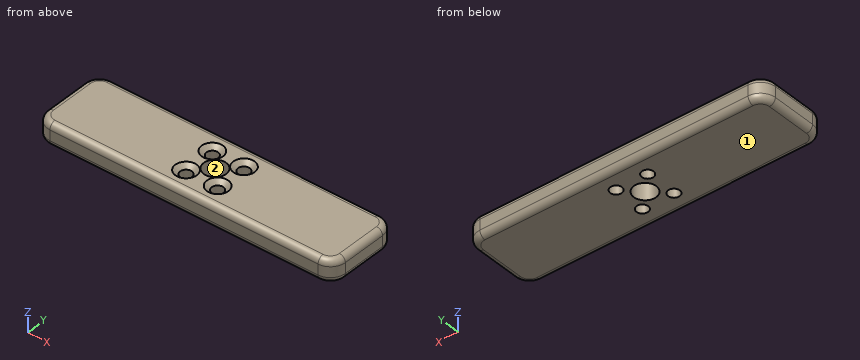
```python
from build123d import *

# Parameters (mm, degrees)
F1_DEPTH        = 9.525
F2_R            = 2.54
F3_R            = 4.7625
F4_DEPTH        = 25.4
F6_D            = 4.9784
F6_CSINK_D      = 9.1186
F6_CSINK_ANGLE  = 100
F6_COPIES_COUNT = 4


# Not quite as in the source:
# - a pattern or mirror of a feature is missing from the dataset's text; its kind, count and spacing are read off the source's solid


with BuildPart() as f1:
    # F0 (on Top) → F1 (new body)
    with BuildSketch(Plane.XY):
        with BuildLine():
            Line((-57.15, -15.875), (57.15, -15.875))
            ThreePointArc((57.15, -15.875), (61.6401280605, -14.0151280605), (63.5, -9.525))
            Line((63.5, -9.525), (63.5, 9.525))
            ThreePointArc((63.5, 9.525), (61.6401280605, 14.0151280605), (57.15, 15.875))
            Line((57.15, 15.875), (-57.15, 15.875))
            ThreePointArc((-57.15, 15.875), (-61.6401280605, 14.0151280605), (-63.5, 9.525))
            Line((-63.5, 9.525), (-63.5, -9.525))
            ThreePointArc((-63.5, -9.525), (-61.6401280605, -14.0151280605), (-57.15, -15.875))
        make_face()
    extrude(amount=F1_DEPTH)

    # F2
    f2_edges = [f1.edges().sort_by_distance(p)[0] for p in [
        (0, -15.875, 9.525),
        (61.640128, -14.015128, 9.525),
        (63.5, 0, 9.525),
        (61.640128, 14.015128, 9.525),
        (0, 15.875, 9.525),
        (-61.640128, 14.015128, 9.525),
        (-63.5, 0, 9.525),
        (-61.640128, -14.015128, 9.525),
        (0, -15.875, 0),
        (61.640128, -14.015128, 0),
        (63.5, 0, 0),
        (61.640128, 14.015128, 0),
        (0, 15.875, 0),
        (-61.640128, 14.015128, 0),
        (-63.5, 0, 0),
        (-61.640128, -14.015128, 0),
    ]]
    fillet(f2_edges, radius=F2_R)

    # F3 (on face) → F4 (cut)
    with BuildSketch(Plane.XY.offset(9.525)):
        Circle(F3_R)
    extrude(amount=-F4_DEPTH, mode=Mode.SUBTRACT)

    # F6 (through all)
    with Locations(Plane.XY.offset(9.525)):
        with Locations((-6.7351920908, 6.7351920908)):
            f6 = CounterSinkHole(F6_D / 2, F6_CSINK_D / 2, counter_sink_angle=F6_CSINK_ANGLE)

    # F6_copies: F6 ×4 about axis
    f6_copies_axis = Axis((0, 0, 0), (0, 0, 1))
    for i in range(1, F6_COPIES_COUNT):
        add(f6.rotate(f6_copies_axis, i * 360 / F6_COPIES_COUNT), mode=Mode.SUBTRACT)


solid = f1.part
```
Could you check a few things on this model? Use its own coordinates, in mm. Face numbers are marked on the shaded views. Coordinates: 2 decimals unless noted, no trailing zeros. Loops run counter-clockwise (first coordinate to the right, second up) from the corner with the lowest first, then second, coordinate; pieces in that order, holes last.
1) Please list where these lines run through material, in increasing order: line 1 along X through (y, z) = (-9, 8); line 2 along X through (y, z) = (9, 2.5); line 3 along Z through (x, y) = (-3, 13.5).
Reported:
line 1: x = -63.29 to -8.28, -5.19 to 5.19, 8.28 to 63.29
line 2: x = -63.5 to -7.77, -5.7 to 5.7, 7.77 to 63.5
line 3: z = 0.01 to 9.52
2) Imagine slicing it at C-C (x = -15). List the corners of the cut face in (y, z) for me (3 decimals).
Reported:
outline: (-15.875, 2.54) arc R2.54 ccw to (-13.335, 0) - (13.335, 0) arc R2.54 ccw to (15.875, 2.54) - (15.875, 6.985) arc R2.54 ccw to (13.335, 9.525) - (-13.335, 9.525) arc R2.54 ccw to (-15.875, 6.985) - close
3) Imagine slicing it at A-A (x = 0). List the corners of the cut face in (y, z) for me (1 decimal), and give its area (3 significant figures).
Reported:
outline: (-15.9, 2.5) arc R2.5 ccw to (-13.3, 0) - (-4.8, 0) - (-4.8, 9.5) - (-13.3, 9.5) arc R2.5 ccw to (-15.9, 7) - close; (4.8, 0) - (13.3, 0) arc R2.5 ccw to (15.9, 2.5) - (15.9, 7) arc R2.5 ccw to (13.3, 9.5) - (4.8, 9.5) - close
area: 206 mm2
4) Imagine slicing it at D-D (z = 5.5). State how many separate pieces and enclosed holes the cut face has, and give its area (3 significant figures).
Reported:
separate pieces: 1
enclosed holes: 5
area: 3,850 mm2
5) Will these pins go through, and if not, where does the flat tip stop? pin 1 Ø5 at (x, z) = (-4, 2) entering from +Y (3 decimals); pin 2 Ø8 at (x, y) = (6.74, 6.74) entering from +Z; pin 3 Ø5.5 at (x, y) = (-6.74, -6.74) entering from +Z.
Reported:
pin 1: stops at y = 15.875
pin 2: stops at z = 9.06
pin 3: stops at z = 8.01
6) Imagine slicing it at B-B (y = 0). List the corners of the cut face in (x, z) for me (1 decimal).
Reported:
outline: (-63.5, 2.5) arc R2.5 ccw to (-61, 0) - (-4.8, 0) - (-4.8, 9.5) - (-61, 9.5) arc R2.5 ccw to (-63.5, 7) - close; (4.8, 0) - (61, 0) arc R2.5 ccw to (63.5, 2.5) - (63.5, 7) arc R2.5 ccw to (61, 9.5) - (4.8, 9.5) - close
7) Thinking about a two-plate mould opening in Y: for the marked faces 1 and 2, which applies, released by +Y, released by -Y, zero draft, split by the parting line, or undercut?
Reported:
face 1: zero draft
face 2: undercut
